```python
from build123d import *

# Parameters (mm, degrees)
SKETCH1_W              = 25
SKETCH1_H              = 10
BASE_PLATE_DEPTH       = 0.79
SKETCH5_R              = 0.79
PIN_HOLDER_DEPTH       = 5
FILLET1_R              = 0.5
SKETCH6_R              = 1
SCREW_HOLES_DEPTH      = 5
SKETCH7_W              = 5
SKETCH7_H              = 0.79
HINGE_GROOVES_DEPTH    = 1.58
FILLET2_R              = 0.5
SKETCH8_R              = 0.4
SKETCH10_W             = 8.42
SKETCH10_H             = 0.79
EXTERNAL_CUTOFF_DEPTH  = 5
SKETCH11_W             = 8.42
SKETCH11_H             = 0.79
EXTERNAL_CUTOFF2_DEPTH = 5


with BuildPart() as part:
    # Sketch1 → Base Plate (new body)
    with BuildSketch(Plane(origin=(0, 0, 0), x_dir=(1, 0, 0), z_dir=(0, 1, 0))):
        with Locations((4.767605634, 0.253521127)):
            Rectangle(SKETCH1_W, SKETCH1_H)
    extrude(amount=BASE_PLATE_DEPTH)

    # Sketch5 → Pin Holder (add)
    with BuildSketch(Plane(origin=(12.267605634, 0, 0), x_dir=(0, 0, -1), z_dir=(1, 0, 0))):
        with BuildLine():
            Line((-3.956478873, 1.58), (-3.956478873, 0.79))
            ThreePointArc((-3.956478873, 0.79), (-4.187864516, 0.231385643), (-4.746478873, 0))
            Line((-4.746478873, 0), (-5.536478873, 0))
            ThreePointArc((-5.536478873, 0), (-6.653707588, 2.697228714), (-3.956478873, 1.58))
        make_face()
        with Locations((-5.536478873, 1.58)):
            Circle(SKETCH5_R, mode=Mode.SUBTRACT)
    pin_holder = extrude(amount=-PIN_HOLDER_DEPTH)

    # Fillet1
    fillet1_edges = [part.edges().sort_by_distance(p)[0] for p in [
        (9.767605634, 0.79, 3.956478873),
    ]]
    fillet(fillet1_edges, radius=FILLET1_R)

    # Sketch6 → Screw Holes (cut)
    with BuildSketch(Plane(origin=(0, 0.79, 0), x_dir=(1, 0, 0), z_dir=(0, 1, 0))):
        with Locations(Location((9.767605634, 1.253521127, 0), (0, 0, 270))):
            Circle(SKETCH6_R)
    screw_holes = extrude(amount=-SCREW_HOLES_DEPTH, mode=Mode.SUBTRACT)

    # Mirror1: Pin Holder, Screw Holes across plane
    add(pin_holder.mirror(Plane(origin=(4.767605634, 0, 0), x_dir=(0, 0, 1), z_dir=(1, 0, 0))))
    add(screw_holes.mirror(Plane(origin=(4.767605634, 0, 0), x_dir=(0, 0, 1), z_dir=(1, 0, 0))), mode=Mode.SUBTRACT)

    # Sketch7 → Hinge Grooves (cut)
    with BuildSketch(Plane.XY.offset(4.746478873)):
        with Locations((14.767605634, 0.395)):
            Rectangle(SKETCH7_W, SKETCH7_H)
        with Locations((4.767605634, 0.395)):
            Rectangle(SKETCH7_W, SKETCH7_H)
        with Locations((-5.232394366, 0.395)):
            Rectangle(SKETCH7_W, SKETCH7_H)
    extrude(amount=-HINGE_GROOVES_DEPTH, mode=Mode.SUBTRACT)

    # Fillet2
    fillet2_edges = [part.edges().sort_by_distance(p)[0] for p in [
        (7.267605634, 0.395, 3.166478873),
        (2.267605634, 0.395, 3.166478873),
    ]]
    fillet(fillet2_edges, radius=FILLET2_R)

    # Wire Groove: sweep along a path in Sketch9
    with BuildLine(Plane.XZ) as wire_groove_path:
        Line((2.767605634, -5.253521127), (2.767605634, 3.166478873))
        Line((2.767605634, 3.166478873), (2.767605634, 3.884059602))
    # Sketch8 → Wire Groove (sweep, cut)
    with BuildSketch(Plane(origin=(0, 0, -5.253521127), x_dir=(-1, 0, 0), z_dir=(0, 0, -1))):
        with Locations((-2.767605634, 0.79)):
            Circle(SKETCH8_R)
    sweep(path=wire_groove_path.line, mode=Mode.SUBTRACT)

    # Sketch10 → External Cutoff (cut)
    with BuildSketch(Plane.ZY.offset(7.732394366)):
        with Locations((-1.043521127, 0.395)):
            Rectangle(SKETCH10_W, SKETCH10_H)
    extrude(amount=-EXTERNAL_CUTOFF_DEPTH, mode=Mode.SUBTRACT)

    # Sketch11 → External Cutoff2 (cut)
    with BuildSketch(Plane(origin=(17.267605634, 0, 0), x_dir=(0, 0, -1), z_dir=(1, 0, 0))):
        with Locations((1.043521127, 0.395)):
            Rectangle(SKETCH11_W, SKETCH11_H)
    extrude(amount=-EXTERNAL_CUTOFF2_DEPTH, mode=Mode.SUBTRACT)


solid = part.part
```
Part model, mm, in its own coordinate system. A direction names the side the tool comes from. Round coordinates to 2 decimals unless told otherwise and drop trailing zeros. Order: outer loops, then holes, each group sorted by start corner. A loop starts at its lowest first (then second) coordinate and runs counter-clockwise, first axis right, second up. Notation, with made-up numbers: M -5,76.25 L 44,76.25 A33 ccw 44,105.25 Z; hole C -10,56 d2. An arc over 180 degrees is marked long. Put each result on its own line as item: value. Start each with the question number.
1. Slice it at D-D on y = 1.85. List the corners of the cut face in (x, z), then the cut area to 3 significant figures.
2. Two-plate mould, pull along X, no slides. Class faces 1 (the face through (2.268, 1.3, 4.6)), 2 (the face through (10.76, 0.4, -1.38)), 3 (the face through (12.268, 0.6, 1.9)), 4 (the face through (5, 0, 0)): +X half, -X half, draft (parallel to the pull), parting line (faces both ways), or undercut.
3. Slice it at A-A on x = 11. List the corners of the cut face in (y, z), then the cut area to 3 significant figures.
4. Slice it at C-C on x = -1. List the corners of the cut face in (y, z), then the cut area to 3 significant figures.
5. Tool access for faces 5 (the face through (7.268, 1.2, 4.6)), 6 (the face through (8, 0.79, -1)), 7 (the face through (2.76, 0.39, -0.88)): list every direction of +Z, -Z, +X, -X, +Y, -Y with a clear straight run to the whole face (end or side of a thin tool).
6. Slice it at B-B on z = 6. List the corners of the cut face in (x, y).
7. Drill centre lines: probe 1 along Z at (x, y) = (2, 1.5); probe 2 along X at (y, z) = (2.55, 6.5); probe 3 along Y at (x, z) = (5, -0.5). Where is each one in solid material? Low to high. Write a range as [from, to].
8. Drop flat-ended pins along their axis: pin 1 (2.5 mm diameter, centred on x = -0.23, z = -1.25, fed in from +Y); pin 2 (0.6 mm diameter, centred on x = 5.5, y = 0, fed in from +Z). Give the stop position or say it passes through.
Findings:
1. outline: M -2.73,3.98 L 2.27,3.98 L 2.27,4.79 L -2.73,4.79 Z; M -2.73,6.28 L 2.27,6.28 L 2.27,7.09 L -2.73,7.09 Z; M 7.27,3.98 L 12.27,3.98 L 12.27,4.79 L 7.27,4.79 Z; M 7.27,6.28 L 12.27,6.28 L 12.27,7.09 L 7.27,7.09 Z
1. area: 16.3 mm2
2. face 1: undercut
2. face 2: undercut
2. face 3: +X half
2. face 4: draft
3. outline: M 0,-5.25 L 0.79,-5.25 L 0.79,3.46 A0.5 cw 1.29,3.96 L 1.58,3.96 A1.58 ccw long 0,5.54 Z; hole C 1.58,5.54 d1.58
3. area: 13.7 mm2
4. outline: M 0,-5.25 L 0.79,-5.25 L 0.79,-1.89 L 0,-1.89 Z; M 0,-0.61 L 0.79,-0.61 L 0.79,3.96 L 1.58,3.96 A1.58 ccw long 0,5.54 Z; hole C 1.58,5.54 d1.58
4. area: 12.7 mm2
5. face 5: +Z, +Y, -Y
5. face 6: -Z, +X, -X, +Y
5. face 7: +Z, -Z, +Y
6. outline: M -2.73,0.07 L 2.27,0.07 L 2.27,0.94 L -2.73,0.94 Z; M -2.73,2.22 L 2.27,2.22 L 2.27,3.09 L -2.73,3.09 Z; M 7.27,0.07 L 12.27,0.07 L 12.27,0.94 L 7.27,0.94 Z; M 7.27,2.22 L 12.27,2.22 L 12.27,3.09 L 7.27,3.09 Z
7. probe 1: [3.96, 4.75], [6.32, 7.11]
7. probe 2: [-2.73, 2.27], [7.27, 12.27]
7. probe 3: [0, 0.79]
8. pin 1: y = 0.79
8. pin 2: z = 3.17
